from build123d import *

# Parameters (mm, degrees)
SKETCH1_R           = 28.011018533
SKETCH1_R_2         = 0.7999984
SKETCH1_R_3         = 0.4499991
SKETCH1_R_4         = 1.49999954
SKETCH1_R_5         = 0.3499993
SKETCH1_R_6         = 0.5499989
BOSS_EXTRUDE1_DEPTH = 1.6
CUT_EXTRUDE1_REACH  = 84.056
SKETCH3_R           = 1.5


with BuildPart() as part:
    # Sketch1 → Boss-Extrude1 (new body)
    with BuildSketch(Plane.XY.offset(3.97256)):
        with Locations((29.99994, 29.99999842)):
            Circle(SKETCH1_R)
        with Locations(Location((43.4299995, 46.7699979, 0), (0, 0, 180))):
            Circle(SKETCH1_R_2, mode=Mode.SUBTRACT)
        with Locations(Location((46.4599401, 16.1399982, 0), (0, 0, 180))):
            Circle(SKETCH1_R_3, mode=Mode.SUBTRACT)
        with Locations(Location((43.4299995, 51.82999794, 0), (0, 0, 180))):
            Circle(SKETCH1_R_2, mode=Mode.SUBTRACT)
        with Locations(Location((43.9199401, 16.1399982, 0), (0, 0, 180))):
            Circle(SKETCH1_R_3, mode=Mode.SUBTRACT)
        with Locations(Location((48.9999401, 16.1399982, 0), (0, 0, 180))):
            Circle(SKETCH1_R_3, mode=Mode.SUBTRACT)
        with Locations(Location((41.3799401, 16.1399982, 0), (0, 0, 180))):
            Circle(SKETCH1_R_3, mode=Mode.SUBTRACT)
        with Locations(Location((38.36999946, 51.82999794, 0), (0, 0, 180))):
            Circle(SKETCH1_R_2, mode=Mode.SUBTRACT)
        with Locations(Location((40.89999948, 49.29999792, 0), (0, 0, 180))):
            Circle(SKETCH1_R_2, mode=Mode.SUBTRACT)
        with Locations(Location((38.36999946, 46.7699979, 0), (0, 0, 180))):
            Circle(SKETCH1_R_2, mode=Mode.SUBTRACT)
        with Locations(Location((38.8399401, 16.1399982, 0), (0, 0, 180))):
            Circle(SKETCH1_R_3, mode=Mode.SUBTRACT)
        with Locations(Location((31.2199401, 16.1399982, 0), (0, 0, 180))):
            Circle(SKETCH1_R_3, mode=Mode.SUBTRACT)
        with Locations(Location((41.3799401, 13.5999982, 0), (0, 0, 180))):
            Circle(SKETCH1_R_3, mode=Mode.SUBTRACT)
        with Locations(Location((43.9199401, 13.5999982, 0), (0, 0, 180))):
            Circle(SKETCH1_R_3, mode=Mode.SUBTRACT)
        with Locations(Location((38.8399401, 13.5999982, 0), (0, 0, 180))):
            Circle(SKETCH1_R_3, mode=Mode.SUBTRACT)
        with Locations(Location((48.9999401, 13.5999982, 0), (0, 0, 180))):
            Circle(SKETCH1_R_3, mode=Mode.SUBTRACT)
        with Locations(Location((46.4599401, 13.5999982, 0), (0, 0, 180))):
            Circle(SKETCH1_R_3, mode=Mode.SUBTRACT)
        with Locations(Location((36.2999401, 16.1399982, 0), (0, 0, 180))):
            Circle(SKETCH1_R_3, mode=Mode.SUBTRACT)
        with Locations(Location((36.2999401, 13.5999982, 0), (0, 0, 180))):
            Circle(SKETCH1_R_3, mode=Mode.SUBTRACT)
        with Locations(Location((33.7599401, 16.1399982, 0), (0, 0, 180))):
            Circle(SKETCH1_R_3, mode=Mode.SUBTRACT)
        with Locations(Location((33.7599401, 13.5999982, 0), (0, 0, 180))):
            Circle(SKETCH1_R_3, mode=Mode.SUBTRACT)
        with Locations(Location((31.2199401, 13.5999982, 0), (0, 0, 180))):
            Circle(SKETCH1_R_3, mode=Mode.SUBTRACT)
        with Locations(Location((29.99994, 29.99999842, 0), (0, 0, 180))):
            Circle(SKETCH1_R_4, mode=Mode.SUBTRACT)
        with Locations(Location((28.6799401, 16.1399982, 0), (0, 0, 180))):
            Circle(SKETCH1_R_3, mode=Mode.SUBTRACT)
        with Locations(Location((26.1399401, 16.1399982, 0), (0, 0, 180))):
            Circle(SKETCH1_R_3, mode=Mode.SUBTRACT)
        with Locations(Location((21.0599401, 16.1399982, 0), (0, 0, 180))):
            Circle(SKETCH1_R_3, mode=Mode.SUBTRACT)
        with Locations(Location((23.5999401, 16.1399982, 0), (0, 0, 180))):
            Circle(SKETCH1_R_3, mode=Mode.SUBTRACT)
        with Locations(Location((18.5199401, 16.1399982, 0), (0, 0, 180))):
            Circle(SKETCH1_R_3, mode=Mode.SUBTRACT)
        with Locations(Location((6.4999997, 32.22499778, 0), (0, 0, 180))):
            Circle(SKETCH1_R_5, mode=Mode.SUBTRACT)
        with Locations(Location((6.4999997, 27.37499986, 0), (0, 0, 180))):
            Circle(SKETCH1_R_5, mode=Mode.SUBTRACT)
        with Locations(Location((3.84999992, 33.42500046, 0), (0, 0, 180))):
            Circle(SKETCH1_R_6, mode=Mode.SUBTRACT)
        with Locations(Location((10.8999401, 16.1399982, 0), (0, 0, 180))):
            Circle(SKETCH1_R_3, mode=Mode.SUBTRACT)
        with Locations(Location((3.84999992, 26.17499718, 0), (0, 0, 180))):
            Circle(SKETCH1_R_6, mode=Mode.SUBTRACT)
        with Locations(Location((21.0599401, 13.5999982, 0), (0, 0, 180))):
            Circle(SKETCH1_R_3, mode=Mode.SUBTRACT)
        with Locations(Location((23.5999401, 13.5999982, 0), (0, 0, 180))):
            Circle(SKETCH1_R_3, mode=Mode.SUBTRACT)
        with Locations(Location((18.5199401, 13.5999982, 0), (0, 0, 180))):
            Circle(SKETCH1_R_3, mode=Mode.SUBTRACT)
        with Locations(Location((28.6799401, 13.5999982, 0), (0, 0, 180))):
            Circle(SKETCH1_R_3, mode=Mode.SUBTRACT)
        with Locations(Location((26.1399401, 13.5999982, 0), (0, 0, 180))):
            Circle(SKETCH1_R_3, mode=Mode.SUBTRACT)
        with Locations(Location((15.9799401, 16.1399982, 0), (0, 0, 180))):
            Circle(SKETCH1_R_3, mode=Mode.SUBTRACT)
        with Locations(Location((15.9799401, 13.5999982, 0), (0, 0, 180))):
            Circle(SKETCH1_R_3, mode=Mode.SUBTRACT)
        with Locations(Location((13.4399401, 16.1399982, 0), (0, 0, 180))):
            Circle(SKETCH1_R_3, mode=Mode.SUBTRACT)
        with Locations(Location((13.4399401, 13.5999982, 0), (0, 0, 180))):
            Circle(SKETCH1_R_3, mode=Mode.SUBTRACT)
        with Locations(Location((10.8999401, 13.5999982, 0), (0, 0, 180))):
            Circle(SKETCH1_R_3, mode=Mode.SUBTRACT)
    extrude(amount=-BOSS_EXTRUDE1_DEPTH)

    # Sketch3 → Cut-Extrude1 (cut, up to next)
    with BuildSketch(Plane.XY.offset(3.97256), mode=Mode.PRIVATE) as cut_extrude1_sk1:
        with Locations((7.483279502, 42.99999842)):
            Circle(SKETCH3_R)
    cut_extrude1_tool1 = extrude(cut_extrude1_sk1.sketch, amount=-CUT_EXTRUDE1_REACH, mode=Mode.PRIVATE) & part.part
    # Sketch3 → Cut-Extrude1 (cut, up to next)
    with BuildSketch(Plane.XY.offset(3.97256), mode=Mode.PRIVATE) as cut_extrude1_sk2:
        with Locations((52.516600498, 42.99999842)):
            Circle(SKETCH3_R)
    cut_extrude1_tool2 = extrude(cut_extrude1_sk2.sketch, amount=-CUT_EXTRUDE1_REACH, mode=Mode.PRIVATE) & part.part
    # Sketch3 → Cut-Extrude1 (cut, up to next)
    with BuildSketch(Plane.XY.offset(3.97256), mode=Mode.PRIVATE) as cut_extrude1_sk3:
        with Locations((29.99994, 3.99999842)):
            Circle(SKETCH3_R)
    cut_extrude1_tool3 = extrude(cut_extrude1_sk3.sketch, amount=-CUT_EXTRUDE1_REACH, mode=Mode.PRIVATE) & part.part
    add(cut_extrude1_tool1.solids().sort_by_distance((7.48328, 42.999998, 3.97256))[0], mode=Mode.SUBTRACT)
    add(cut_extrude1_tool2.solids().sort_by_distance((52.5166, 42.999998, 3.97256))[0], mode=Mode.SUBTRACT)
    add(cut_extrude1_tool3.solids().sort_by_distance((29.99994, 3.999998, 3.97256))[0], mode=Mode.SUBTRACT)


solid = part.part
Work out the finished part from the listing and answer in its coordinate system (mm). Coordinates: 2 decimals unless noted, no trailing zeros. Write each loop counter-clockwise with the first axis right and the second up, starting at its lowest first coordinate (ties: lowest second). Pieces come first, ordered by that corner, then holes. Notation, with made-up numbers: M -29.75,76.25 L 9.25,76.25 A21 cw 9.25,102.25 Z; hole C 70,66.5 d7. An arc over 180 degrees is marked long. Write item = value, one per line.
1. The part is cut by section A-A (z = 3.7). State how many separate pieces and enclosed holes the cut face has, then the cut area to 3 significant figures.
Solution:
separate_pieces = 1
enclosed_holes = 45
area = 2,400 mm2
2. The part is cut by section B-B (y = 35). Determine the outline of the cut face in (x, z).
Solution:
outline = M 2.44,2.37 L 57.56,2.37 L 57.56,3.97 L 2.44,3.97 Z
3. The part is cut by section C-C (y = 20). Determine the outline of the cut face in (x, z).
Solution:
outline = M 3.83,2.37 L 56.17,2.37 L 56.17,3.97 L 3.83,3.97 Z
4. Straight lines are drawn through the part: line 1 (Y direction, x = 16, z = 2.55); line 2 (Y direction, x = 24, z = 2.7); line 3 (Y direction, x = 29, z = 3.15). For each, find the intervals that lie inside material, in ascending order. Write a range as from..to.
Solution:
line_1 = 5.74..13.15, 14.05..15.69, 16.59..54.26
line_2 = 2.64..13.39, 13.81..15.93, 16.35..57.36
line_3 = 2.01..2.88, 5.12..13.28, 13.92..15.82, 16.46..28.88, 31.12..57.99
5. Determine the mould class of faces 1 (the face through (7.77, 12.96, 3.18)), 2 (the face through (36, 30, 2.373)), 3 (the face through (7.288, 44.487, 3.184)) for opening direction Y: released by +Y, released by -Y, zero draft, split by the parting line, or undercut.
Solution:
face_1 = split by the parting line
face_2 = zero draft
face_3 = undercut
6. A flat-ended cylindrical pin translates along its axis: pin 1 (0.7 mm diameter, centred on x = 3.85, y = 26.17, fed in from -Z). Find the tip coordinate at first contact, or state that the pin passes through.
Solution:
pin_1 = through
